Could you check a few things on this drawing? It's one solid part, dimensions in mm from its lowest x, y, z. A direction names the side the tool comes from. Give positions to 0.01 mm unless a question says otherwise; leave off trailing zeros. Loops run counter-clockwise (first coordinate to the right, second up) from the corner with the lowest first, then second, coordinate; pieces in that order, holes last. Notation, with made-up numbers: M -40,-35 L 7,-35 A14 cw 7,-23 Z; hole C 15,81 d5. An arc over 180 degrees is marked long. Answer in a Markdown table with one row per item. Add a question column.
1. I need wall thicknesses on line 1 along Z through (x, y) = (6, 5.05); line 2 along X through (y, z) = (4.9, 33); line 3 along Z through (x, y) = (7, 4.8). Which ranges of each line are inside material? Lowest first, please. Write a range as from..to.
2. If we section it at C-C on x = 17.5: List the corners of the cut face in (y, z) for me, then the cut area to 3 significant figures.
3. Which directions (+Z, -Z, +X, -X, +Y, -Y) give clear straight access to the entire face, cutting with the end or side of a thin tool? Please do the marked faces 1, 2 and 3.
4. I'm going to push flat-ended pins straight in: pin 1 Ø1.7 at (y, z) = (5, 8.5) entering from -X; pin 2 Ø1 at (y, z) = (5, 10) entering from +X; pin 3 Ø2.5 at (x, z) = (6, 21) entering from +Y; pin 4 Ø1.5 at (y, z) = (1.5, 11) entering from +X. Where does each tip first touch, or does it pass through?
5. If we section it at B-B on z = 33: List the corners of the cut face in (x, y) for me.
6. If we section it at A-A on x = 32: List the corners of the cut face in (y, z) for me, then the cut area to 3 significant figures.
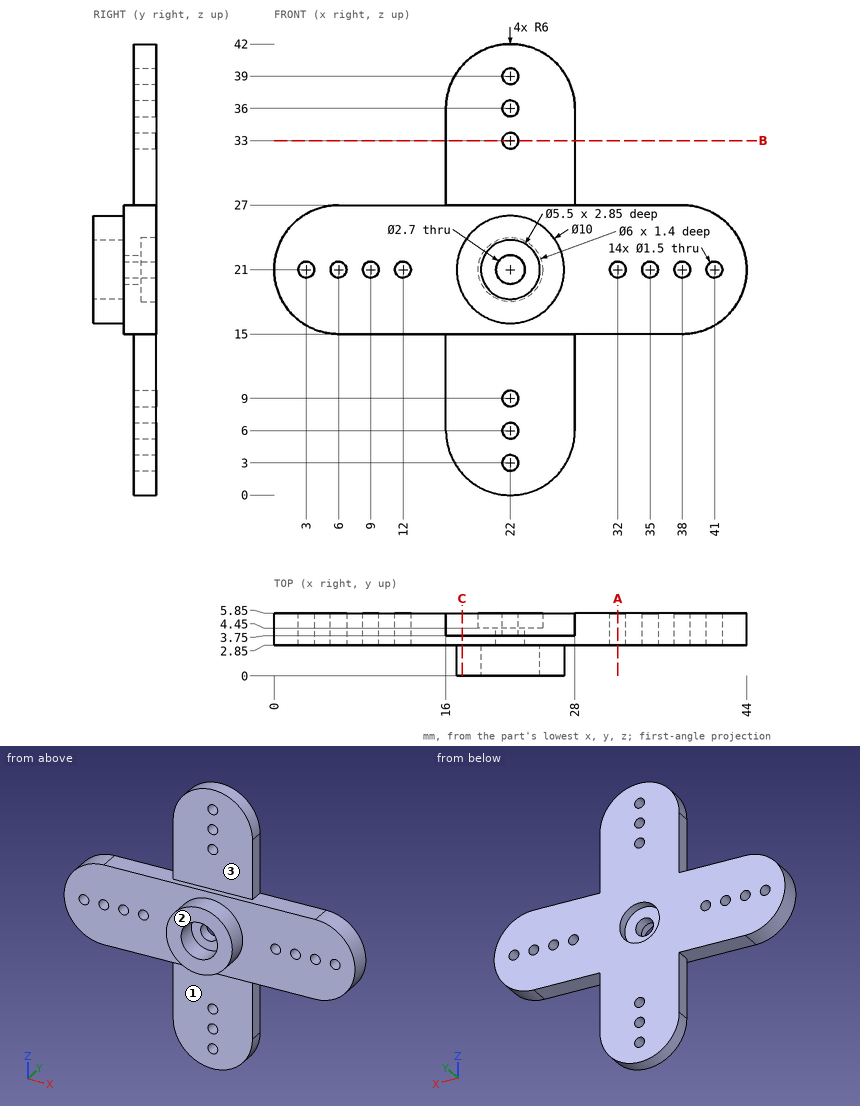
Results:
| question | item | result |
|---|---|---|
| 1 | line 1 | 15..20.25, 21.75..27 |
| 1 | line 2 | 16..21.25, 22.75..28 |
| 1 | line 3 | 15..27 |
| 2 | outline | M 0,18.82 L 2.85,18.82 L 2.85,15 L 3.75,15 L 3.75,2.03 L 5.85,2.03 L 5.85,39.97 L 3.75,39.97 L 3.75,27 L 2.85,27 L 2.85,23.18 L 0,23.18 Z |
| 2 | area | 103 mm2 |
| 3 | face 1 | -Z, +X, -X, -Y |
| 3 | face 2 | +Z, -Z, +X, -X, -Y |
| 3 | face 3 | +Z, +X, -X, -Y |
| 4 | pin 1 | x = 16 |
| 4 | pin 2 | x = 28 |
| 4 | pin 3 | y = 5.85 |
| 4 | pin 4 | through |
| 5 | outline | M 16,3.75 L 21.25,3.75 L 21.25,5.85 L 16,5.85 Z; M 22.75,3.75 L 28,3.75 L 28,5.85 L 22.75,5.85 Z |
| 6 | outline | M 2.85,15 L 5.85,15 L 5.85,20.25 L 2.85,20.25 Z; M 2.85,21.75 L 5.85,21.75 L 5.85,27 L 2.85,27 Z |
| 6 | area | 31.5 mm2 |
